Input: part model. Units: mm. Frame: model coordinates. A direction names the side the tool comes from. Round coordinates to 2 decimals unless told otherwise and drop trailing zeros. Loops run counter-clockwise (first coordinate to the right, second up) from the corner with the lowest first, then second, coordinate; pieces in that order, holes last. Notation, with made-up numbers: M -3,-4 L 10,-4 A37 ccw 10,34 Z; hole C -8.5,10 d3. An arc over 180 degrees is marked long. Return JSON: item names as keys, results as strings. Group by question number.
1) Contact query for flat-ended pins moving along their axis: P1, Ø10, axis at x = -11, z = 19, coming from the +Y side; P2, Ø5, axis at x = -1, y = -1.5, coming from the +Z side; P3, Ø5, axis at y = -4, z = 19, coming from the +X side; P4, Ø11, axis at x = 0, y = 0, coming from the -Z side. Output: stop coordinate, or through.
2) Access query for faces 4 (the face through (-0.34, -1.55, 12.24)), 5 (the face through (2, 0, 24.191)). Directions: +Z, -Z, +X, -X, +Y, -Y. A direction counts if a zero-diameter tool reaches every point of the face in a straight line with its end or side. Return the directions, or none.
3) Material intervals for line 1 (Y direction, x = 0, z = 42.75); line 2 (Y direction, x = 0, z = 31); line 3 (Z direction, x = 36, y = 26), sorted ascending. Write a range as from..to.
4) Mould query, pull axis X, two halves, no side actions, for faces 1 (the face through (12.2, -5.06, 41.34)), 2 (the face through (-3.78, -2.9, 37.07)), 3 (the face through (-11, -9, 32.855)). Classes: +X half, -X half, draft (parallel to the pull), parting line (faces both ways), or undercut.
5) Section C-C (z = 38). Output: boundary loops of the cut face in (x, y) (1 decimal), plus the area to 3 significant figures.
6) Section D-D (z = 15). Output: boundary loops of the cut face in (x, y) (1 decimal).
7) Section A-A (x = 0). Output: boundary loops of the cut face in (y, z).
from build123d import *

# Parameters (mm, degrees)
F2_R     = 4.7625
F4_DEPTH = 25.4
F5_R     = 1.5875
F6_DEPTH = 25.4


with BuildPart() as f1:
    # F0 (on Front) → F1 (revolve)
    with BuildSketch(Plane.XZ):
        Polygon((0, 24.795596), (0, 0), (44.45, 17.542299), (44.45, 24.795596), align=None)
        Polygon((0, 49.591192), (0, 24.795596), (44.45, 24.795596), (44.45, 32.854902), (13.208, 32.854902), (13.208, 49.591192), align=None)
    revolve(axis=Axis((0, 0, 24.795596), (0, 0, 1)))

    # F2 (on face) → F4 (cut)
    with BuildSketch(Plane.XY.offset(49.591192)):
        Circle(F2_R)
    extrude(amount=-F4_DEPTH, mode=Mode.SUBTRACT)

    # F5 (on Top) → F6 (cut)
    with BuildSketch(Plane.XY):
        Circle(F5_R)
    extrude(amount=F6_DEPTH, mode=Mode.SUBTRACT)


solid = f1.part
Returned:
{
 "1": {"P1": "stops at y = 44.04", "P2": "stops at z = 24.19", "P3": "stops at x = 44.42", "P4": "stops at z = 0.63"},
 "2": {"face 4": "+Z, -Z", "face 5": "+Z"},
 "3": {"line 1": "y = -13.21..-4.76, 4.76..13.21", "line 2": "y = -44.45..-4.76, 4.76..44.45", "line 3": "z = 17.53..32.85"},
 "4": {"face 1": "parting line", "face 2": "undercut", "face 3": "draft"},
 "5": {"outline": "C 0,0 d26.4; hole C 0,0 d9.5", "area": "477 mm^2"},
 "6": {"outline": "C 0,0 d76; hole C 0,0 d3.2"},
 "7": {"outline": "M -44.45,17.54 L -1.59,0.63 L -1.59,24.19 L -4.76,24.19 L -4.76,49.59 L -13.21,49.59 L -13.21,32.85 L -44.45,32.85 Z; M 1.59,0.63 L 44.45,17.54 L 44.45,32.85 L 13.21,32.85 L 13.21,49.59 L 4.76,49.59 L 4.76,24.19 L 1.59,24.19 Z"}
}
